Job drawing, mm, ordinate dimensions from the low corner. One solid piece. Give positions to 0.01 mm unless a question says otherwise; leave off trailing zeros. Loops run counter-clockwise (first coordinate to the right, second up) from the corner with the lowest first, then second, coordinate; pieces in that order, holes last. Notation, with made-up numbers: (66, -25.75) - (88, -25.75) arc R19 ccw to (88, -6.75) - close; hole circle Ø11 at (69, 13.5). An arc over 180 degrees is marked (long way). Use a Markdown table: item, result.
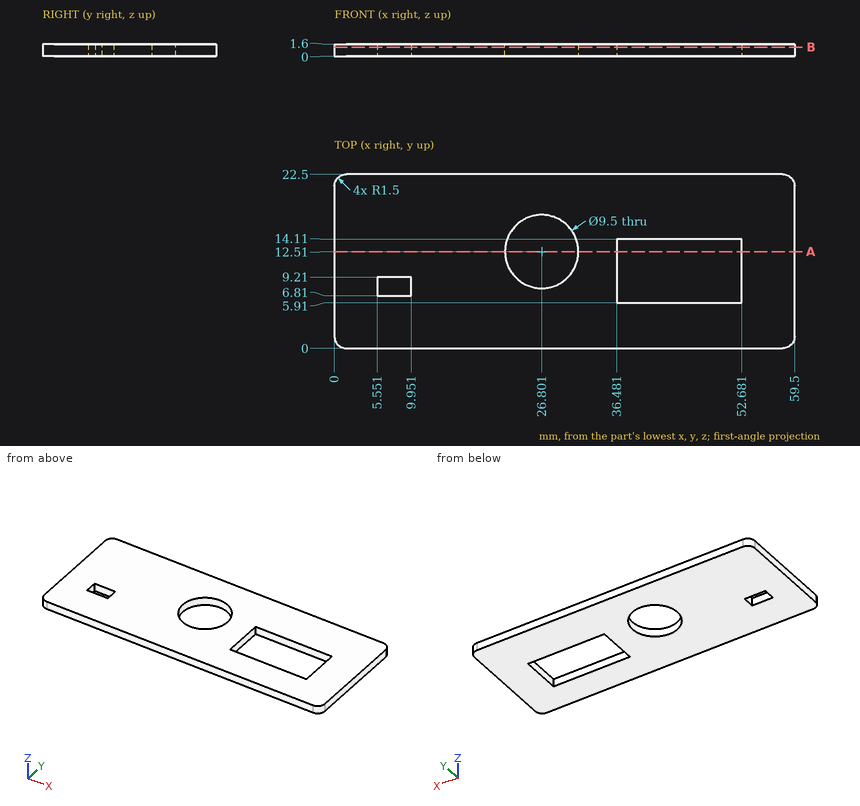
(1) Pin check, flat tip, straight feed: P1, Ø5.5, axis at x = 26.801, y = 12.51, coming from the +Z side. Stop position of the tip, or through.
Computed:
| item | result |
|---|---|
| P1 | through |
(2) Slice it at B-B, the plane z = 1.2. Write the cut outline in (x, y).
Computed:
| item | result |
|---|---|
| outline | (0, 1.5) arc R1.5 ccw to (1.5, 0) - (58, 0) arc R1.5 ccw to (59.5, 1.5) - (59.5, 21) arc R1.5 ccw to (58, 22.5) - (1.5, 22.5) arc R1.5 ccw to (0, 21) - close; hole (5.55, 6.81) - (9.95, 6.81) - (9.95, 9.21) - (5.55, 9.21) - close; hole circle Ø9.5 at (26.8, 12.51); hole (36.48, 5.91) - (52.68, 5.91) - (52.68, 14.11) - (36.48, 14.11) - close |
(3) Drill centre lines: probe 1 along Y at (x, z) = (50.5, 1); probe 2 along Y at (x, z) = (8, 0.3); probe 3 along X at (y, z) = (6, 1.4). Where is each one in solid material? Low to high. Write a range as [from, to].
Computed:
| item | result |
|---|---|
| probe 1 | [0, 5.91], [14.11, 22.5] |
| probe 2 | [0, 6.81], [9.21, 22.5] |
| probe 3 | [0, 36.48], [52.68, 59.5] |
(4) Slice it at A-A, the plane y = 12.51. Write the cut outline in (x, z).
Computed:
| item | result |
|---|---|
| outline | (0, 0) - (22.05, 0) - (22.05, 1.6) - (0, 1.6) - close; (31.55, 0) - (36.48, 0) - (36.48, 1.6) - (31.55, 1.6) - close; (52.68, 0) - (59.5, 0) - (59.5, 1.6) - (52.68, 1.6) - close |
